Autodesk Inventor part; units mm, degrees
ref_plane "YZ Plane" through (0, 0, 0) normal (1, 0, 0) x (0, 1, 0)
ref_plane "XZ Plane" through (0, 0, 0) normal (0, 1, 0) x (-1, 0, 0)
ref_plane "XY Plane" through (0, 0, 0) normal (0, 0, 1) x (1, 0, 0)
sketch "Блок1" plane through (0, 0, 0) normal (0, 0, 1) x (1, 0, 0)
  line L0 (-20.8941, 6.9119) -> (-9.8941, 6.9119)
  line L1 (-8.8941, 8.4119) -> (-6.8941, 8.4119)
  point P0 (-11.6441, 7.6619)
sketch "Эскиз1" plane through (0, 0, 0) normal (0, 0, 1) x (1, 0, 0)
  line L0 (0.0239, 0.0663) -> (10.8239, 0.0663)
  line L1 (14.0239, 3.2663) -> (14.0239, 3.5663)
  arc A0 (10.8239, 0.0663) -> (14.0239, 3.2663) centre (10.8239, 3.2663) ccw
  line L2 (0.0239, 0.0663) -> (0.0239, 2.0663)
  line L3 (12.0239, 3.0663) -> (12.0239, 3.5663)
  arc A1 (11.0239, 2.0663) -> (12.0239, 3.0663) centre (11.0239, 3.0663) ccw
  line L4 (14.0239, 3.5663) -> (14.0239, 5.0663)
  line L5 (0.0239, 5.0663) -> (7.906, 5.0663)
  line L6 (0.0239, 2.0663) -> (11.0239, 2.0663)
  line L7 (12.0239, 3.5663) -> (14.0239, 3.5663)
  point P0 (0, 0)
  point P1 (14.0239, 0.0663)
  point P2 (11.0239, 2.0663)
  dimension "d8" = 2
  dimension "d15" = 3.2
  dimension "d18" = 5
  dimension "d19" = 10.8
revolve "Вращение1" add sketch "Эскиз1" angle 360 about axis through (0.0239, 5.0663, 0) along (1, 0, 0)
properties part number "12"
Design review of the part built by this model. Coordinates are the model's own, in mm. Round coordinates to 2 decimals unless told otherwise and drop trailing zeros. Write each loop counter-clockwise with the first axis right and the second up, starting at its lowest first coordinate (ties: lowest second). Pieces come first, ordered by that corner, then holes.
Item 1: Clearance check with flat-ended pins moving along their axes: pin 1 Ø1.5 at (x, z) = (9.5, 0.5) entering from -Y; pin 2 Ø1.2 at (y, z) = (6, 1) entering from -X; pin 3 Ø1 at (x, y) = (4.5, 7) entering from -Z. State where each tip first meets the part, or that it passes through.
Item 2: For probe 1 along Y at (x, z) = (4, 0); probe 2 along Z at (x, y) = (1.5, 4.25); probe 3 along Z at (x, y) = (2.5, 2.5), list the stretches that pass through material, from the lowest coordinate up.
Item 3: We need section A-A on x = 2.5. Write out the cut boundary in (y, z).
Item 4: The part is to be moulded in two halves that separate along Z. For faces 1 (the cylindrical face through (5.601, 2.205, -0.901)), 2 (the cylindrical face through (5.5, 0.297, -1.502)), 3 (the flat face through (0.024, 5.1, 3.3)), say which applies: +Z half, -Z half, draft (parallel to the pull), parting line (faces both ways), or undercut.
Returned:
1. pin 1: stops at y = 0.07
1. pin 2: stops at x = 12.02
1. pin 3: stops at z = -4.79
2. probe 1: y = 0.07 to 2.07, 8.07 to 10.07
2. probe 2: z = -4.93 to -2.89, 2.89 to 4.93
2. probe 3: z = -4.29 to -1.55, 1.55 to 4.29
3. outline: circle Ø10 at (5.07, 0); hole circle Ø6 at (5.07, 0)
4. face 1: undercut
4. face 2: parting line
4. face 3: draft
